Here's how the part is built. I have some questions about the finished solid (model axes, mm). Give positions to 0.01 mm unless a question says otherwise; leave off trailing zeros. Order: outer loops, then holes, each group sorted by start corner. A loop starts at its lowest first (then second) coordinate and runs counter-clockwise, first axis right, second up. Notation, with made-up numbers: M 14.5,-19.75 L 48.5,-19.75 A14 ccw 48.5,-3.75 Z; hole C 39.5,-20.75 d10. An arc over 180 degrees is marked long. Use CSV: the item, a comma, the result in double quotes. Start each with the question number.
```python
from build123d import *

# Parameters (mm, degrees)
SKETCH1_W           = 150
SKETCH1_H           = 100
BOSS_EXTRUDE1_DEPTH = 3
SKETCH2_R           = 1.425
CUT_EXTRUDE1_DEPTH  = 10
LPATTERN1_COUNT     = 2
LPATTERN1_PITCH     = 76
SKETCH5_R           = 1.6
CUT_EXTRUDE4_DEPTH  = 10
SKETCH6_R           = 1.425
CUT_EXTRUDE5_DEPTH  = 10


with BuildPart() as part:
    # Sketch1 → Boss-Extrude1 (new body)
    with BuildSketch(Plane(origin=(0, 0, 0), x_dir=(1, 0, 0), z_dir=(0, 1, 0))):
        Rectangle(SKETCH1_W, SKETCH1_H)
    extrude(amount=BOSS_EXTRUDE1_DEPTH)

    # Sketch2 → Cut-Extrude1 (cut)
    with BuildSketch(Plane(origin=(0, 3, 0), x_dir=(1, 0, 0), z_dir=(0, 1, 0))):
        with Locations((-63, 38)):
            Circle(SKETCH2_R)
    cut_extrude1 = extrude(amount=-CUT_EXTRUDE1_DEPTH, mode=Mode.SUBTRACT)

    # LPattern1: Cut-Extrude1 ×2
    with Locations(*[(0, 0, i * LPATTERN1_PITCH) for i in range(1, LPATTERN1_COUNT)]):
        add(cut_extrude1, mode=Mode.SUBTRACT)

    # Sketch5 → Cut-Extrude4 (cut)
    with BuildSketch(Plane(origin=(0, 3, 0), x_dir=(1, 0, 0), z_dir=(0, 1, 0))):
        with Locations((-34.7, 32.4)):
            Circle(SKETCH5_R)
        with Locations((-6.8, 32.4)):
            Circle(SKETCH5_R)
        with Locations((-1.7, -20)):
            Circle(SKETCH5_R)
        with Locations((-50, -18.4)):
            Circle(SKETCH5_R)
    extrude(amount=-CUT_EXTRUDE4_DEPTH, mode=Mode.SUBTRACT)

    # Sketch6 → Cut-Extrude5 (cut)
    with BuildSketch(Plane.XZ):
        with Locations((63, 38)):
            Circle(SKETCH6_R)
        with Locations((63, -38)):
            Circle(SKETCH6_R)
    extrude(amount=-CUT_EXTRUDE5_DEPTH, mode=Mode.SUBTRACT)


solid = part.part
```
Q1. Imagine slicing it at A-A, the plane z = -32.4. Please give me the cut outline in (x, y).
Q2. Imagine slicing it at B-B, the plane x = -50. Please give me the cut outline in (y, z).
Q3. We'd pull the mould along X, two halves only. Please class faces 1 (the face through (-75, 1, 1)), 2 (the face through (-1.908, 1.521, 18.414)), 3 (the face through (-1, 3, -1)): pulls with the +X half, pulls with the -X half, needs draft (parallel to the pull), parting line crosses it, or undercut.
Q4. For P1, Ø3.5, axis at x = -1.7, z = 20, coming from the -Y side; P2, Ø3, axis at x = -34.7, z = -32.4, coming from the +Y side, each with a flat end and sliding along its axis, tell me the tip position at first contact or that it passes through.
Q5. I need wall thicknesses on line 1 (Z direction, x = 63, y = 0.75) (3 decimals); line 2 (X direction, y = 1.8, z = -32.4); line 3 (Z direction, x = -6.8, y = 2.1). Which ranges of each line are inside material? Lowest first, please. Write a range as [from, to].
Reply:
1,outline,"M -75,0 L -36.3,0 L -36.3,3 L -75,3 Z; M -33.1,0 L -8.4,0 L -8.4,3 L -33.1,3 Z; M -5.2,0 L 75,0 L 75,3 L -5.2,3 Z"
2,outline,"M 0,-50 L 3,-50 L 3,16.8 L 0,16.8 Z; M 0,20 L 3,20 L 3,50 L 0,50 Z"
3,face 1,"pulls with the -X half"
3,face 2,"undercut"
3,face 3,"needs draft"
4,P1,"stops at y = 0"
4,P2,"passes through"
5,line 1,"z = [-50, -39.425], [-36.575, 36.575], [39.425, 50]"
5,line 2,"x = [-75, -36.3], [-33.1, -8.4], [-5.2, 75]"
5,line 3,"z = [-50, -34], [-30.8, 50]"
